```python
from build123d import *

# Parameters (mm, degrees)
F1_DEPTH = 4.2
F2_W     = 20.9
F2_H     = 4.1
F3_DEPTH = 10
F5_DEPTH = 4.1
F6_W     = 0.9
F6_H     = 2
F7_DEPTH = 0.1
F9_DEPTH = 25


with BuildPart() as f1:
    # F0 (on Top) → F1 (new body)
    with BuildSketch(Plane.XY):
        with BuildLine():
            Line((0, 10.05713), (-8.199971, 10.05713))
            Line((-8.199971, 10.05713), (-10.55, 5.35))
            Line((-10.55, 5.35), (-10.55, -4.15))
            Line((-10.55, -4.15), (-6.896709, -5.343926))
            ThreePointArc((-6.896709, -5.343926), (-6.589984, -5.417979), (-6.275429, -5.44287))
            Line((-6.275429, -5.44287), (-6.046804, -5.44287))
            ThreePointArc((-6.046804, -5.44287), (-5.653998, -5.403917), (-5.276493, -5.288574))
            Line((-5.276493, -5.288574), (-1.155466, -3.56865))
            ThreePointArc((-1.155466, -3.56865), (0, -3.337205), (1.155466, -3.56865))
            Line((1.155466, -3.56865), (5.276493, -5.288574))
            ThreePointArc((5.276493, -5.288574), (5.653998, -5.403917), (6.046804, -5.44287))
            Line((6.046804, -5.44287), (6.275429, -5.44287))
            ThreePointArc((6.275429, -5.44287), (6.589984, -5.417979), (6.896709, -5.343926))
            Line((6.896709, -5.343926), (10.55, -4.15))
            Line((10.55, -4.15), (10.55, 5.35))
            Line((10.55, 5.35), (8.199971, 10.05713))
            Line((8.199971, 10.05713), (0, 10.05713))
        make_face()
    extrude(amount=F1_DEPTH)

    # F2 (on face) → F3 (cut)
    with BuildSketch(Plane.XZ.offset(5.44287)):
        with Locations((0, 2.05)):
            Rectangle(F2_W, F2_H)
    extrude(amount=-F3_DEPTH, mode=Mode.SUBTRACT)

    # F4 (on face) → F5 (cut)
    with BuildSketch(Plane(origin=(0, 0, 0), x_dir=(1, 0, 0), z_dir=(0, 0, -1))):
        Polygon((10.45, -4.55713), (-10.45, -4.55713), (-10.45, -5.35), (-8.156886, -9.943129), (8.15174, -9.953437), (10.45, -5.35), align=None)
    extrude(amount=-F5_DEPTH, mode=Mode.SUBTRACT)

    # F6 (on Top) → F7 (join)
    with BuildSketch(Plane.XY):
        with Locations((-11, 4.25713)):
            Rectangle(F6_W, F6_H)
        with Locations((-11, 1.15713)):
            Rectangle(F6_W, F6_H)
        with Locations((11, 1.15713)):
            Rectangle(F6_W, F6_H)
        with Locations((11, 4.25713)):
            Rectangle(F6_W, F6_H)
    extrude(amount=F7_DEPTH)

    # F8 (on face) → F9 (cut)
    with BuildSketch(Plane.XY.offset(4.2)):
        with BuildLine():
            ThreePointArc((-3.33593, 2.273972), (-2.369798, 3.275535), (-2.017699, 4.621852))
            ThreePointArc((-2.017699, 4.621852), (-6.114016, 7.019753), (-6.199468, 2.273972))
            ThreePointArc((-6.199468, 2.273972), (-4.767699, 1.871852), (-3.33593, 2.273972))
        make_face()
        with BuildLine():
            ThreePointArc((-3.33593, 2.273972), (-4.767699, 1.871852), (-6.199468, 2.273972))
            Line((-6.199468, 2.273972), (-6.199468, -1.400822))
            Line((-6.199468, -1.400822), (-3.222397, -1.400822))
            Line((-3.222397, -1.400822), (-3.33593, 2.273972))
        make_face()
        with BuildLine():
            ThreePointArc((6.199468, 2.273972), (7.165601, 3.275535), (7.517699, 4.621852))
            ThreePointArc((7.517699, 4.621852), (3.421383, 7.019753), (3.33593, 2.273972))
            ThreePointArc((3.33593, 2.273972), (4.767699, 1.871852), (6.199468, 2.273972))
        make_face()
        with BuildLine():
            ThreePointArc((6.199468, 2.273972), (4.767699, 1.871852), (3.33593, 2.273972))
            Line((3.33593, 2.273972), (3.222397, -1.400822))
            Line((3.222397, -1.400822), (6.199468, -1.400822))
            Line((6.199468, -1.400822), (6.199468, 2.273972))
        make_face()
    extrude(amount=-F9_DEPTH, mode=Mode.SUBTRACT)


solid = f1.part
```
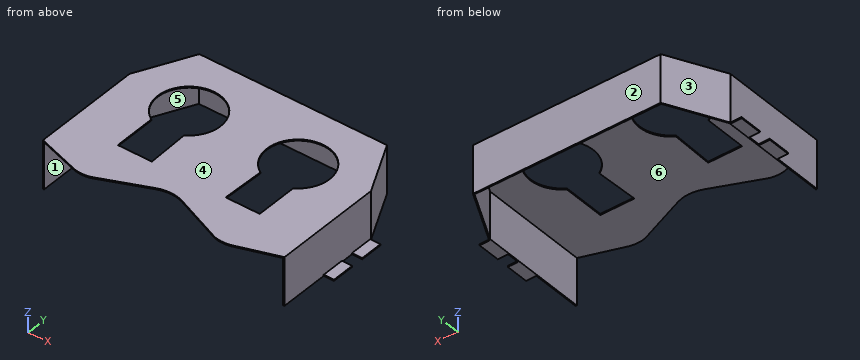
The listing builds one solid part. Answer for the finished solid, in the listing's coordinates (mm). Face numbers are marked on the shaded views. A direction names the side the tool comes from. Give positions to 0.01 mm unless a question says otherwise; leave off trailing zeros. Loops run counter-clockwise (first coordinate to the right, second up) from the corner with the lowest first, then second, coordinate; pieces in that order, holes last. Notation, with made-up numbers: M -20,10 L 16,10 A30 ccw 16,34 Z; hole C 82.25,-9 d10. An arc over 180 degrees is marked long. One line per item, written item: value.
Q1. A cutting plane is placed at B-B on y = 1. Determine the outline of the cut face in (x, z).
Working result:
outline: M -11.45,0 L -10.45,0 L -10.45,4.1 L -6.2,4.1 L -6.2,4.2 L -10.55,4.2 L -10.55,0.1 L -11.45,0.1 Z; M -3.3,4.1 L 3.3,4.1 L 3.3,4.2 L -3.3,4.2 Z; M 6.2,4.1 L 10.45,4.1 L 10.45,0 L 11.45,0 L 11.45,0.1 L 10.55,0.1 L 10.55,4.2 L 6.2,4.2 Z
Q2. Find the intervals of material crossed by line 1 (Y direction, x = -8.25, z = 0.7); line 2 (Y direction, x = -8.75, z = 1.3), in increasing order. Write a range as from..to.
Working result:
line 1: y = 9.76..9.96
line 2: y = 8.76..8.96
Q3. A cutting plane is placed at C-C on y = -1.75. Determine the outline of the cut face in (x, z), then the cut area to 3 significant figures.
Working result:
outline: M -10.55,0 L -10.45,0 L -10.45,4.1 L 10.45,4.1 L 10.45,0 L 10.55,0 L 10.55,4.2 L -10.55,4.2 Z
area: 2.93 mm^2
Q4. A flat-ended cylindrical pin translates along its axis: P1, Ø1.5, axis at x = -1.5, y = 5, coming from the -Z side. Find the tip coordinate at first contact, or state that the pin passes through.
Working result:
P1: stops at z = 4.1
Q5. A cutting plane is placed at A-A on z = 1.6. Determine the outline of the cut face in (x, y), then the cut area to 3 significant figures.
Working result:
outline: M -10.55,-4.15 L -10.45,-4.18 L -10.45,5.35 L -8.16,9.94 L 8.15,9.95 L 10.45,5.35 L 10.45,-4.18 L 10.55,-4.15 L 10.55,5.35 L 8.2,10.06 L -8.2,10.06 L -10.55,5.35 Z
area: 4.61 mm^2
Q6. Determine the mould class of the marked faces 3, 4, 5 and 6 for opening direction X: +X half, -X half, draft (parallel to the pull), parting line (faces both ways), or undercut.
Working result:
face 3: -X half
face 4: draft
face 5: undercut
face 6: undercut
Q7. A cutting plane is placed at D-D on x = 9.75. Determine the outline of the cut face in (y, z).
Working result:
outline: M -4.41,4.1 L 6.75,4.1 L 6.75,0 L 6.95,0 L 6.95,4.2 L -4.41,4.2 Z
Q8. For the marked faces 1 and 2, determine the directions among +Z, -Z, +X, -X, +Y, -Y from which every point of the face is accessible in a straight line to the end or side of a thin tool.
Working result:
face 1: -Z, -Y
face 2: +Z, -Z, +X, -X, +Y
